Input: part model. Units: mm. Frame: model coordinates. Face numbers are marked on the shaded views. A direction names the side the tool comes from. Coordinates: 2 decimals unless noted, no trailing zeros. Loops run counter-clockwise (first coordinate to the right, second up) from the corner with the lowest first, then second, coordinate; pieces in that order, holes last.
(1) Section D-D, the plane y = -6. Return loops of the section in (x, z).
(2) Contact query for flat-ended pins moving along their axis: P1, Ø8.5, axis at x = -24.5, z = 15.5, coming from the +Y side; P2, Ø8, axis at y = 8.5, z = -20, coming from the +X side; P3, Ø8, axis at x = -20.5, z = 6, coming from the -Y side; P4, Ø8, axis at x = -22, y = 0, coming from the +Z side. Output: stop coordinate, or through.
(3) Line query: L1, parallel to Z at x = -20, y = -12; L2, parallel to Z at x = -20.2, y = -5.5; L3, parallel to Z at x = -23, y = 15.5. Output: solid intervals per line, ascending.
(4) Set-up query: the marked faces 4, 5 and 6. Return all of +Z, -Z, +X, -X, +Y, -Y with unobstructed straight access to the full face (end or side cutting, diameter ignored); none if empty.
(5) Section C-C, the plane z = -27. Return loops of the section in (x, y), then the cut area to 3 significant figures.
(6) Mould query, pull axis Y, two halves, no side actions, for the marked faces 1, 2 and 3. Classes: released by +Y, released by -Y, zero draft, split by the parting line, or undercut.
(7) Section A-A, the plane x = 0. Return loops of the section in (y, z), then the cut area to 3 significant figures.
(8) Section B-B, the plane y = -15. Return loops of the section in (x, z), then the cut area to 3 significant figures.
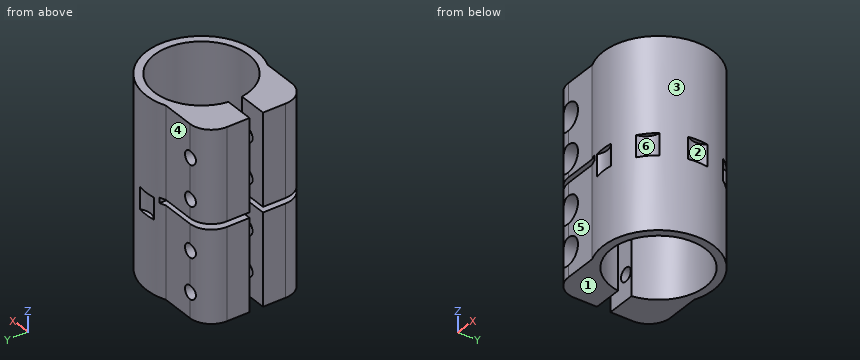
```python
from build123d import *

# Parameters (mm, degrees)
F1_DEPTH       = 35
F3_D           = 5
F3_START       = 1.8205079
F3_CBORE_D     = 10
F3_CBORE_DEPTH = 8
F4_W           = 22.4
F4_H           = 2
F5_DEPTH       = 27.5
F6_R           = 6
F7_DEPTH       = 8


with BuildPart() as f1:
    # F0 (on Top) → F1 (new body, symmetric)
    with BuildSketch(Plane.XY):
        with BuildLine():
            ThreePointArc((-17.3192642082, 2.5086026559), (17.5, 0), (-17.3192642082, -2.5086026559))
            Line((-17.3192642082, -2.5086026559), (-28.1192642082, -2.5086026559))
            Line((-28.1192642082, -2.5086026559), (-28.1192642082, -10.9086026559))
            ThreePointArc((-28.1192642082, -10.9086026559), (-25.7761184577, -16.5654569054), (-20.1192642082, -18.9086026559))
            Line((-20.1192642082, -18.9086026559), (-7.9192642082, -18.9086026559))
            ThreePointArc((-7.9192642082, -18.9086026559), (20.5, 0), (-7.9192642082, 18.9086026559))
            Line((-7.9192642082, 18.9086026559), (-20.1192642082, 18.9086026559))
            ThreePointArc((-20.1192642082, 18.9086026559), (-25.7761184577, 16.5654569054), (-28.1192642082, 10.9086026559))
            Line((-28.1192642082, 10.9086026559), (-28.1192642082, 2.5086026559))
            Line((-28.1192642082, 2.5086026559), (-17.3192642082, 2.5086026559))
        make_face()
    extrude(amount=F1_DEPTH, both=True)

    # F3 (through all)
    # its depths count from where the whole tool has entered the part; down to there all is cleared
    with Locations(Plane.XZ.offset(18.9086026559).offset(-F3_START)):
        with Locations((-20.2, -25.683545606), (-20.2, -10.683545606), (-20.2, 7.816454394), (-20.2, 22.816454394)):
            CounterBoreHole(F3_D / 2, F3_CBORE_D / 2, F3_CBORE_DEPTH)

    # F4 (on Front) → F5 (cut, symmetric)
    with BuildSketch(Plane.XZ):
        with Locations((-16.9192642082, 0)):
            Rectangle(F4_W, F4_H)
    extrude(amount=F5_DEPTH, both=True, mode=Mode.SUBTRACT)

    # F6 (on Top) → F7 (cut)
    with BuildSketch(Plane.XY):
        with Locations((0, -25)):
            Circle(F6_R)
        with Locations((17.6776695297, -17.6776695297)):
            Circle(F6_R)
        with Locations((25, 0)):
            Circle(F6_R)
        with Locations((17.6776695297, 17.6776695297)):
            Circle(F6_R)
        with Locations((0, 25)):
            Circle(F6_R)
    extrude(amount=-F7_DEPTH, mode=Mode.SUBTRACT)


solid = f1.part
```
Report:
1. outline: (-28.12, -35) - (-16.44, -35) - (-16.44, -1) - (-28.12, -1) - close; (-28.12, 1) - (-16.44, 1) - (-16.44, 35) - (-28.12, 35) - close; (16.44, -35) - (19.6, -35) - (19.6, 35) - (16.44, 35) - close; hole circle Ø5 at (-20.2, -25.68); hole circle Ø5 at (-20.2, -10.68); hole circle Ø5 at (-20.2, 7.82); hole circle Ø5 at (-20.2, 22.82)
2. P1: stops at y = 18.91
2. P2: stops at x = 20
2. P3: stops at y = -18.91
2. P4: stops at z = 35
3. L1: z = -35 to -30.68, -20.69 to -15.68, -5.69 to -1, 1 to 2.82, 12.81 to 17.82, 27.81 to 35
3. L2: z = -35 to -28.18, -23.18 to -13.18, -8.18 to -1, 1 to 5.32, 10.32 to 20.32, 25.32 to 35
3. L3: z = -35 to -1, 1 to 35
4. face 4: +Z, -Z, -X, +Y
4. face 5: +Z, -Z, -X, -Y
4. face 6: +X, -Y
5. outline: (-28.12, -10.91) arc R8 ccw to (-25.02, -17.23) - (-25.02, -9.09) - (-22.33, -9.09) - (-22.33, -2.51) - (-28.12, -2.51) - close; (-28.12, 2.51) - (-22.33, 2.51) - (-22.33, 18.6) arc R8 ccw to (-28.12, 10.91) - close; (-18.07, -9.09) - (-15.38, -9.09) - (-15.38, -18.91) - (-7.92, -18.91) arc R20.5 ccw (long way) to (-7.92, 18.91) - (-18.07, 18.91) - (-18.07, 2.51) - (-17.32, 2.51) arc R17.5 cw (long way) to (-17.32, -2.51) - (-18.07, -2.51) - close
5. area: 508 mm2
6. face 1: zero draft
6. face 2: undercut
6. face 3: split by the parting line
7. outline: (-20.5, -35) - (-17.5, -35) - (-17.5, 35) - (-20.5, 35) - (-20.5, 0) - (-19, 0) - (-19, -8) - (-20.5, -8) - close; (17.5, -35) - (20.5, -35) - (20.5, -8) - (19, -8) - (19, 0) - (20.5, 0) - (20.5, 35) - (17.5, 35) - close
7. area: 396 mm2
8. outline: (-26.99, -35) - (-9.01, -35) - (-9.01, -1) - (-26.99, -1) - close; (-26.99, 1) - (-9.01, 1) - (-9.01, 35) - (-26.99, 35) - close; (9.01, -35) - (13.97, -35) - (13.97, -8) - (12.31, -8) - (12.31, 0) - (13.97, 0) - (13.97, 35) - (9.01, 35) - close; hole circle Ø10 at (-20.2, -25.68); hole circle Ø10 at (-20.2, -10.68); hole circle Ø10 at (-20.2, 7.82); hole circle Ø10 at (-20.2, 22.82)
8. area: 1,240 mm2
